from build123d import *

# Parameters (mm, degrees)
F1_DEPTH = 12.7
F3_DEPTH = 10.16
F4_W     = 6.35
F4_H     = 177.1998706725
F5_DEPTH = 6.35


with BuildPart() as f1:
    # F0 (on Front) → F1 (new body)
    with BuildSketch(Plane.XZ):
        with BuildLine():
            Line((0, 88.9), (0, 18.9734820172))
            ThreePointArc((0, 18.9734820172), (5.0506124764, 3.7727442912), (18.1938919224, -5.3828725206))
            Line((18.1938919224, -5.3828725206), (311.3668292683, -92.1214634146))
            ThreePointArc((311.3668292683, -92.1214634146), (461.1537705997, -16.2686651285), (355.6, 114.3))
            Line((355.6, 114.3), (25.4, 114.3))
            ThreePointArc((25.4, 114.3), (7.4394877579, 106.8605122421), (0, 88.9))
        make_face()
    extrude(amount=F1_DEPTH)

    # F2 (on face) → F3 (join)
    with BuildSketch(Plane.XZ.offset(12.7)):
        with BuildLine():
            ThreePointArc((25.4, 114.3), (7.4394877579, 106.8605122421), (0, 88.9))
            Line((0, 88.9), (425.1607648032, 88.9))
            ThreePointArc((425.1607648032, 88.9), (392.6265445323, 107.751368334), (355.6, 114.3))
            Line((355.6, 114.3), (25.4, 114.3))
        make_face()
    extrude(amount=F3_DEPTH)

    # F4 (on face) → F5 (join)
    with BuildSketch(Plane.XZ.offset(12.7)):
        Polygon((76.2, 88.9), (69.85, 88.9), (69.85, -20.6659271787), (76.2, -22.5446478313), align=None)
        Polygon((152.4, 88.9), (146.05, 88.9), (146.05, -43.2105750099), (152.4, -45.0892956626), align=None)
        Polygon((228.6, 88.9), (222.25, 88.9), (222.25, -65.7552228412), (228.6, -67.6339434938), align=None)
        with Locations((301.625, 0.3000646637)):
            Rectangle(F4_W, F4_H)
        Polygon((381, 88.9), (374.65, 88.9), (374.65, -99.9058233698), (381, -98.5692189258), align=None)
    extrude(amount=F5_DEPTH)


solid = f1.part
Geometry: final body of the model. Coordinates: model frame, mm. A direction names the side the tool comes from. Give positions to 0.01 mm unless a question says otherwise; leave off trailing zeros. Write each loop counter-clockwise with the first axis right and the second up, starting at its lowest first coordinate (ties: lowest second). Pieces come first, ordered by that corner, then holes. Notation, with made-up numbers: (60.5, -13.75) - (83.5, -13.75) arc R23 ccw to (83.5, 17.25) - close; hole circle Ø2 at (-27, 79.5). An arc over 180 degrees is marked (long way). Return JSON: item names as keys, results as strings. Group by question number.
1) First-contact query: P1, Ø3, axis at y = -3, z = 91.5, coming from the +X side; P2, Ø7, axis at x = 149, z = 3.5, coming from the -Y side; P3, Ø5, axis at y = -16.5, z = -21, coming from the -X side. Flat tips, straight axial feed; report the tip coordinate or a pass-through.
2) Mould query, pull axis X, two halves, no side actions, for faces 1 (the flat face through (210, -18, 88.9)), 2 (the flat face through (413, -12.7, -4)), 3 (the cylindrical face through (4.91, -6.26, 3.96)). Classes: released by +X, released by -X, zero draft, split by the parting line, or undercut.
3) Set-up query: faces 4 (the cylindrical face through (7.64, -11.27, 107.06)), 5 (the flat face through (187, -12.7, 13)), 6 (the flat face through (34, -12.7, 35)). Return all of +Z, -Z, +X, -X, +Y, -Y with unobstructed straight access to the full face (end or side cutting, diameter ignored); none if empty.
4) Section B-B on x = 292. Return the cut outline in (y, z), plus the area to 3 significant figures.
5) Section A-A on z = 24. Return the cut outline in (x, y), plus the area to 3 significant figures.
6) Line query: line 1 (X direction, y = -14, z = 10.5); line 2 (X direction, y = -15.75, z = -43); line 3 (Y direction, x = 434.5, z = 28.5). Output: solid intervals per line, ascending.
7) Section D-D on z = 53. Return the cut outline in (x, y), plus the area to 3 significant figures.
8) Section C-C on y = -8.5. Return the cut outline in (x, z).
Filled in:
{
 "1": {"P1": "stops at x = 423.83", "P2": "stops at y = -19.05", "P3": "stops at x = 69.85"},
 "2": {"face 1": "undercut", "face 2": "zero draft", "face 3": "released by -X"},
 "3": {"face 4": "+Z, -X, +Y, -Y", "face 5": "-Z, -Y", "face 6": "-Z, -X, -Y"},
 "4": {"outline": "(-22.86, 88.9) - (-12.7, 88.9) - (-12.7, -86.39) - (0, -86.39) - (0, 114.3) - (-22.86, 114.3) - close", "area": "2,810 mm^2"},
 "5": {"outline": "(0, -12.7) - (69.85, -12.7) - (69.85, -19.05) - (76.2, -19.05) - (76.2, -12.7) - (146.05, -12.7) - (146.05, -19.05) - (152.4, -19.05) - (152.4, -12.7) - (222.25, -12.7) - (222.25, -19.05) - (228.6, -19.05) - (228.6, -12.7) - (298.45, -12.7) - (298.45, -19.05) - (304.8, -19.05) - (304.8, -12.7) - (374.65, -12.7) - (374.65, -19.05) - (381, -19.05) - (381, -12.7) - (462.1, -12.7) - (462.1, 0) - (0, 0) - close", "area": "6,070 mm^2"},
 "6": {"line 1": "x = 69.85 to 76.2, 146.05 to 152.4, 222.25 to 228.6, 298.45 to 304.8, 374.65 to 381", "line 2": "x = 146.05 to 152.4, 222.25 to 228.6, 298.45 to 304.8, 374.65 to 381", "line 3": "y = -12.7 to 0"},
 "7": {"outline": "(0, -12.7) - (69.85, -12.7) - (69.85, -19.05) - (76.2, -19.05) - (76.2, -12.7) - (146.05, -12.7) - (146.05, -19.05) - (152.4, -19.05) - (152.4, -12.7) - (222.25, -12.7) - (222.25, -19.05) - (228.6, -19.05) - (228.6, -12.7) - (298.45, -12.7) - (298.45, -19.05) - (304.8, -19.05) - (304.8, -12.7) - (374.65, -12.7) - (374.65, -19.05) - (381, -19.05) - (381, -12.7) - (452.95, -12.7) - (452.95, 0) - (0, 0) - close", "area": "5,950 mm^2"},
 "8": {"outline": "(0, 18.97) arc R25.4 ccw to (18.19, -5.38) - (311.37, -92.12) arc R107.95 ccw (long way) to (355.6, 114.3) - (25.4, 114.3) arc R25.4 ccw to (0, 88.9) - close"}
}
